The model under review builds one solid part; all positions refer to its coordinate system, in mm. Round coordinates to 2 decimals unless told otherwise and drop trailing zeros. Answer as a JSON object with one key per item and string values. Group by question number.
1. Clearance check with flat-ended pins moving along their axes: P1, Ø5, axis at x = -1.5, y = 65.5, coming from the +Z side; P2, Ø1.5, axis at y = 94, z = 89, coming from the +X side; P3, Ø4, axis at x = 10.5, z = 110, coming from the -Y side. State where each tip first meets the part, or that it passes through.
2. Mouldability with a two-part tool opening along X and no side actions: class faces 1 (the face through (-11.923, 15.21, 53.692)), 2 (the face through (50.076, 15.21, -15.77)), 3 (the face through (-49, 0, -20)) as released by +X, released by -X, zero draft, split by the parting line, or undercut.
3. To check wall thickness, follow probe 1 along X at (y, z) = (10, 0); probe 2 along Y at (x, z) = (48, 126.5). State the ranges of each line that lie inside material, in increasing order. Write a range as [from, to].
```python
from build123d import *

# Parameters (mm, degrees)
F0_R   = 55
F0_R_2 = 52.5


with BuildPart() as f2:
    # F2: sweep along a path in F1
    with BuildLine(Plane.YZ) as f2_path:
        Line((0, 0), (30, 0))
        ThreePointArc((30, 0), (114.852814, 35.147186), (150, 120))
        Line((150, 120), (150, 150))
    # F0 (on Front) → F2 (sweep)
    with BuildSketch(Plane.XZ):
        Circle(F0_R)
        Circle(F0_R_2, mode=Mode.SUBTRACT)
    sweep(path=f2_path.line)


solid = f2.part
```
Recorded:
{
 "1": {"P1": "stops at z = 67.24", "P2": "stops at x = 26.6", "P3": "stops at y = 94.76"},
 "2": {"face 1": "split by the parting line", "face 2": "undercut", "face 3": "zero draft"},
 "3": {"probe 1": "x = [-55, -52.5], [52.5, 55]", "probe 2": "y = [123.15, 128.73], [171.27, 176.85]"}
}
